```python
from build123d import *

# Parameters (mm, degrees)
SKETCH1_R           = 88.9
BOSS_EXTRUDE1_DEPTH = 6.35
SKETCH2_R           = 50.8
CUT_EXTRUDE1_DEPTH  = 7.35
FILLET2_R           = 4.826
SKETCH3_R           = 6.35
CUT_EXTRUDE2_DEPTH  = 7.35


with BuildPart() as part:
    # Sketch1 → Boss-Extrude1 (new body)
    with BuildSketch(Plane(origin=(0, 0, 0), x_dir=(1, 0, 0), z_dir=(0, 1, 0))):
        Circle(SKETCH1_R)
    extrude(amount=BOSS_EXTRUDE1_DEPTH)

    # Sketch2 → Cut-Extrude1 (cut, through all)
    with BuildSketch(Plane(origin=(0, 6.35, 0), x_dir=(1, 0, 0), z_dir=(0, 1, 0))):
        Circle(SKETCH2_R)
    extrude(amount=-CUT_EXTRUDE1_DEPTH, mode=Mode.SUBTRACT)

    # Fillet2
    fillet2_edges = [part.edges().sort_by_distance(p)[0] for p in [
        (-50.8, 6.35, 0),
    ]]
    fillet(fillet2_edges, radius=FILLET2_R)

    # Sketch3 → Cut-Extrude2 (cut, through all)
    with BuildSketch(Plane.XZ):
        with Locations((0, -79.375)):
            Circle(SKETCH3_R)
        with Locations((79.375, 0)):
            Circle(SKETCH3_R)
        with Locations((-79.375, 0)):
            Circle(SKETCH3_R)
        with Locations((0, 79.375)):
            Circle(SKETCH3_R)
    extrude(amount=-CUT_EXTRUDE2_DEPTH, mode=Mode.SUBTRACT)


solid = part.part
```
CAD build for the part. Positions are in the model's coordinates, mm. Coordinates: 2 decimals unless noted, no trailing zeros. Write each loop counter-clockwise with the first axis right and the second up, starting at its lowest first coordinate (ties: lowest second). Pieces come first, ordered by that corner, then holes. Notation, with made-up numbers: (25, 45) -> (29, 45) arc R11 ccw to (29, 63) -> close; hole circle Ø5 at (-32, -37.5). An arc over 180 degrees is marked (long way). Return JSON: item names as keys, results as strings. Group by question number.
Q1. Drill centre lines: line 1 (Z direction, x = 0, y = 0.75) (3 decimals); line 2 (X direction, y = 1, z = -3); line 3 (Z direction, x = 0, y = 3.75) (3 decimals). Where is each one in solid material? Low to high.
Q2. Cut at D-D, the plane x = 64. Give the cut face in (y, z), then the cut area to 3 significant figures.
Q3. Pull direction Z, two halves, no side cores. Call faces 1 (the face through (84.795, 3.131, -26.703)), 2 (the face through (-1.377, 3.131, -85.574)), 3 (the face through (-41, 6.35, 38)): released by +Z, released by -Z, zero draft, split by the parting line, or undercut.
Q4. Cut at A-A, the plane z = 0. Give the cut face in (x, y) (3 decimals), then the cut area to 3 significant figures.
Q5. Cut at B-B, the plane x = 0. Give the cut face in (y, z) (3 decimals), then the cut area to 3 significant figures.
Q6. Cut at C-C, the plane y = 2.75. Give the cut face in (x, z) (3 decimals).
Q7. Flat gauge pins, fed straight in: pin 1 (3 mm diameter, centred on y = 0.5, z = 61.5, fed in from +X); pin 2 (11.5 mm diameter, centred on x = 0, z = 79.375, fed in from +Y); pin 3 (1.5 mm diameter, centred on y = 1.5, z = 38, fed in from +X). Where does each tip first touch, or does it go through?
Returned:
{
 "1": {"line 1": "z = -88.9 to -85.725, -73.025 to -50.8, 50.8 to 73.025, 85.725 to 88.9", "line 2": "x = -88.85 to -84.97, -73.78 to -50.71, 50.71 to 73.78, 84.97 to 88.85", "line 3": "z = -88.9 to -85.725, -73.025 to -51.344, 51.344 to 73.025, 85.725 to 88.9"},
 "2": {"outline": "(0, -61.7) -> (6.35, -61.7) -> (6.35, 61.7) -> (0, 61.7) -> close", "area": "784 mm2"},
 "3": {"face 1": "split by the parting line", "face 2": "undercut", "face 3": "zero draft"},
 "4": {"outline": "(-88.9, 0) -> (-85.725, 0) -> (-85.725, 6.35) -> (-88.9, 6.35) -> close; (-73.025, 0) -> (-50.8, 0) -> (-50.8, 1.524) arc R4.826 ccw to (-55.626, 6.35) -> (-73.025, 6.35) -> close; (50.8, 0) -> (73.025, 0) -> (73.025, 6.35) -> (55.626, 6.35) arc R4.826 ccw to (50.8, 1.524) -> close; (85.725, 0) -> (88.9, 0) -> (88.9, 6.35) -> (85.725, 6.35) -> close", "area": "313 mm2"},
 "5": {"outline": "(0, -88.9) -> (6.35, -88.9) -> (6.35, -85.725) -> (0, -85.725) -> close; (0, -73.025) -> (6.35, -73.025) -> (6.35, -55.626) arc R4.826 ccw to (1.524, -50.8) -> (0, -50.8) -> close; (0, 50.8) -> (1.524, 50.8) arc R4.826 ccw to (6.35, 55.626) -> (6.35, 73.025) -> (0, 73.025) -> close; (0, 85.725) -> (6.35, 85.725) -> (6.35, 88.9) -> (0, 88.9) -> close", "area": "313 mm2"},
 "6": {"outline": "circle Ø177.8 at (0, 0); hole circle Ø12.7 at (-79.375, 0); hole circle Ø101.917 at (0, 0); hole circle Ø12.7 at (0, -79.375); hole circle Ø12.7 at (0, 79.375); hole circle Ø12.7 at (79.375, 0)"},
 "7": {"pin 1": "stops at x = 65.6", "pin 2": "passes through", "pin 3": "stops at x = 80.72"}
}
